```python
from build123d import *

# Parameters (mm, degrees)
SKETCH2_R           = 2
BOSS_EXTRUDE1_DEPTH = 25
SKETCH4_R           = 74.5
SKETCH4_R_2         = 72.4
CUT_EXTRUDE1_DEPTH  = 3
FILLET1_R           = 3


with BuildPart() as part:
    # Sketch1 → Revolve-Thin1 (revolve)
    with BuildSketch(Plane.XY, mode=Mode.PRIVATE) as revolve_thin1_sk:
        with BuildLine():
            ThreePointArc((-70, 0), (-74.393398282, 19.393398282), (-86.715728753, 35))
            Line((-86.715728753, 35), (-87.972807475, 33.444444444))
            ThreePointArc((-87.972807475, 33.444444444), (-76.198136136, 18.53146947), (-72, 0))
            Line((-72, 0), (-70, 0))
        make_face()
    revolve(revolve_thin1_sk.sketch.rotate(Axis((0, 0, 0), (0, 1, 0)), 270), axis=Axis((0, 0, 0), (0, 1, 0)))

    # Sketch2 → Boss-Extrude1 (add)
    # profile 1 of 4: a face of its own
    with BuildSketch(Plane(origin=(0, 25, 0), x_dir=(-1, 0, 0), z_dir=(0, -1, 0))):
        with BuildLine():
            ThreePointArc((3.8828898, -68.960815695), (2.829681089, -77.845605343), (4, -86.715728753))
            Line((4, -86.715728753), (-4, -86.715728753))
            ThreePointArc((-4, -86.715728753), (-2.829681089, -77.845605343), (-3.8828898, -68.960815695))
            ThreePointArc((-3.8828898, -68.960815695), (0, -64), (3.8828898, -68.960815695))
        make_face()
        with Locations(Location((0, -68, 0), (0, 0, 90))):
            Circle(SKETCH2_R, mode=Mode.SUBTRACT)
    # profile 2 of 4: a face of its own
    with BuildSketch(Plane(origin=(0, 25, 0), x_dir=(-1, 0, 0), z_dir=(0, -1, 0))):
        with BuildLine():
            ThreePointArc((68.960815695, 3.8828898), (77.845605343, 2.829681089), (86.715728753, 4))
            Line((86.715728753, 4), (86.715728753, -4))
            ThreePointArc((86.715728753, -4), (77.845605343, -2.829681089), (68.960815695, -3.8828898))
            ThreePointArc((68.960815695, -3.8828898), (64, 0), (68.960815695, 3.8828898))
        make_face()
        with Locations(Location((68, 0, 0), (0, 0, 90))):
            Circle(SKETCH2_R, mode=Mode.SUBTRACT)
    # profile 3 of 4: a face of its own
    with BuildSketch(Plane(origin=(0, 25, 0), x_dir=(-1, 0, 0), z_dir=(0, -1, 0))):
        with BuildLine():
            ThreePointArc((-3.8828898, 68.960815695), (-2.829681089, 77.845605343), (-4, 86.715728753))
            Line((-4, 86.715728753), (4, 86.715728753))
            ThreePointArc((4, 86.715728753), (2.829681089, 77.845605343), (3.8828898, 68.960815695))
            ThreePointArc((3.8828898, 68.960815695), (0, 64), (-3.8828898, 68.960815695))
        make_face()
        with Locations(Location((0, 68, 0), (0, 0, 90))):
            Circle(SKETCH2_R, mode=Mode.SUBTRACT)
    # profile 4 of 4: a face of its own
    with BuildSketch(Plane(origin=(0, 25, 0), x_dir=(-1, 0, 0), z_dir=(0, -1, 0))):
        with BuildLine():
            ThreePointArc((-86.624516405, 3.976275972), (-86.692922667, 1.988661001), (-86.715728753, 0))
            ThreePointArc((-86.715728753, 0), (-86.692922667, -1.988661001), (-86.624516405, -3.976275972))
            ThreePointArc((-86.624516405, -3.976275972), (-77.798482599, -2.829401113), (-68.960815695, -3.8828898))
            ThreePointArc((-68.960815695, -3.8828898), (-64, 0), (-68.960815695, 3.8828898))
            ThreePointArc((-68.960815695, 3.8828898), (-77.798482599, 2.829401113), (-86.624516405, 3.976275972))
        make_face()
        with Locations(Location((-68, 0, 0), (0, 0, 90))):
            Circle(SKETCH2_R, mode=Mode.SUBTRACT)
    extrude(amount=BOSS_EXTRUDE1_DEPTH)

    # Sketch3 → Cut-Revolve1 (revolve, cut)
    with BuildSketch(Plane.XY, mode=Mode.PRIVATE) as cut_revolve1_sk:
        with BuildLine():
            Line((-72, 0), (-99.127196695, 0))
            Line((-99.127196695, 0), (-99.127196695, 33.444444444))
            Line((-99.127196695, 33.444444444), (-87.972807475, 33.444444444))
            ThreePointArc((-87.972807475, 33.444444444), (-76.198136136, 18.53146947), (-72, 0))
        make_face()
    revolve(cut_revolve1_sk.sketch.rotate(Axis((0, 0, 0), (0, 1, 0)), 270), axis=Axis((0, 0, 0), (0, 1, 0)), mode=Mode.SUBTRACT)

    # Sketch4 → Cut-Extrude1 (cut)
    with BuildSketch(Plane(origin=(0, 25, 0), x_dir=(1, 0, 0), z_dir=(0, 1, 0))):
        Circle(SKETCH4_R)
        Circle(SKETCH4_R_2, mode=Mode.SUBTRACT)
    extrude(amount=-CUT_EXTRUDE1_DEPTH, mode=Mode.SUBTRACT)

    # Fillet1
    fillet1_edges = [part.edges().sort_by_distance(p)[0] for p in [
        (-74.5, 25, 0),
        (0, 25, 74.5),
        (74.5, 25, 0),
        (0, 25, -74.5),
    ]]
    fillet(fillet1_edges, radius=FILLET1_R - 0.0001)  # a hair under: the kernel refuses the full size


solid = part.part
```
Geometry: final body of the model. Coordinates: model frame, mm. A direction names the side the tool comes from. Give positions to 0.01 mm unless a question says otherwise; leave off trailing zeros. Order: outer loops, then holes, each group sorted by start corner. A loop starts at its lowest first (then second) coordinate and runs counter-clockwise, first axis right, second up. Notation, with made-up numbers: (82.25, 81) -> (94.25, 81) arc R16 ccw to (94.25, 106) -> close; hole circle Ø7 at (9, -34.5). An arc over 180 degrees is marked (long way). Write each question's results on one line, items separated by ' | '. Start each with the question number.
1) First-contact query: pin 1 (10 mm diameter, centred on x = 23, y = 26.5, fed in from -Z); pin 2 (4.5 mm diameter, centred on x = 0, z = 68, fed in from +Y); pin 3 (0.7 mm diameter, centred on x = -74, z = 0, fed in from +Y); pin 4 (2.5 mm diameter, centred on x = 0.5, z = 68.5, fed in from +Y). Flat tips, straight axial feed; report the tip coordinate or a pass-through.
2) Line query: line 1 (Z direction, x = -68, y = 17.5); line 2 (X direction, y = 12, z = 0); line 3 (X direction, y = 7, z = -43). Output: solid intervals per line, ascending. Write a range as from..to.
3) Set-up query: faces 1 (the flat face through (-0.3, 0, -64.3)), 2 (the flat face through (70, 25, -1)). Return all of +Z, -Z, +X, -X, +Y, -Y with unobstructed straight access to the full face (end or side cutting, diameter ignored); none if empty.
4) Section B-B (y = 17.5). Return loops of the section in (x, z), then the cut area to 3 significant figures.
5) Section A-A (y = 5.5). Return loops of the section in (x, z), then the cut area to 3 significant figures.
Calculated:
1) pin 1: z = -82.75 | pin 2: y = 25 | pin 3: y = 22 | pin 4: through
2) line 1: -33.31..-28.01, -4..-2, 2..4, 28.01..33.31 | line 2: -73.71..-70, -66..-64, 64..66, 70..73.71 | line 3: -58.46..-55.93, 55.93..58.46
3) face 1: +Z, -Z, +X, -X, -Y | face 2: +Y
4) outline: circle Ø151.44 at (0, 0); hole (-73.48, -3.07) arc R73.54 ccw to (-3.07, -73.48) arc R36 ccw to (-3.88, -68.96) arc R4 cw (long way) to (3.88, -68.96) arc R36 ccw to (3.07, -73.48) arc R73.54 ccw to (73.48, -3.07) arc R36 ccw to (68.96, -3.88) arc R4 cw (long way) to (68.96, 3.88) arc R36 ccw to (73.48, 3.07) arc R73.54 ccw to (3.07, 73.48) arc R36 ccw to (3.88, 68.96) arc R4 cw (long way) to (-3.88, 68.96) arc R36 ccw to (-3.07, 73.48) arc R73.54 ccw to (-73.48, 3.07) arc R36 ccw to (-68.96, 3.88) arc R4 cw (long way) to (-68.96, -3.88) arc R36 ccw to start; hole circle Ø4 at (-68, 0); hole circle Ø4 at (0, -68); hole circle Ø4 at (0, 68); hole circle Ø4 at (68, 0) | area: 1,230 mm2
5) outline: circle Ø144.71 at (0, 0); hole (-70.25, -3.59) arc R70.34 ccw to (-3.59, -70.25) arc R36 ccw to (-3.88, -68.96) arc R4 cw (long way) to (3.88, -68.96) arc R36 ccw to (3.59, -70.25) arc R70.34 ccw to (70.25, -3.59) arc R36 ccw to (68.96, -3.88) arc R4 cw (long way) to (68.96, 3.88) arc R36 ccw to (70.25, 3.59) arc R70.34 ccw to (3.59, 70.25) arc R36 ccw to (3.88, 68.96) arc R4 cw (long way) to (-3.88, 68.96) arc R36 ccw to (-3.59, 70.25) arc R70.34 ccw to (-70.25, 3.59) arc R36 ccw to (-68.96, 3.88) arc R4 cw (long way) to (-68.96, -3.88) arc R36 ccw to start; hole circle Ø4 at (-68, 0); hole circle Ø4 at (0, -68); hole circle Ø4 at (0, 68); hole circle Ø4 at (68, 0) | area: 1,020 mm2
